```python
from build123d import *

# Parameters (mm, degrees)
F0_W      = 400
F0_H      = 500
F1_DEPTH  = 3
F2_W      = 10
F2_H      = 3
F2_W_2    = 20
F3_DEPTH  = 3
F4_W      = 20
F4_H      = 3
F5_DEPTH  = 3.001
F6_W      = 300
F6_H      = 300
F7_DEPTH  = 25
F8_R      = 25
F9_R      = 3
F10_DEPTH = 25


with BuildPart() as f1:
    # F0 (on Right) → F1 (new body)
    with BuildSketch(Plane.YZ):
        Rectangle(F0_W, F0_H)
    extrude(amount=F1_DEPTH)

    # F2 (on face) → F3 (join, through all)
    with BuildSketch(Plane.YZ.offset(3)):
        with Locations((-195, 251.5)):
            Rectangle(F2_W, F2_H)
        with Locations((-160, 251.5)):
            Rectangle(F2_W_2, F2_H)
        with Locations((-120, 251.5)):
            Rectangle(F2_W_2, F2_H)
        with Locations((-80, 251.5)):
            Rectangle(F2_W_2, F2_H)
        with Locations((-40, 251.5)):
            Rectangle(F2_W_2, F2_H)
        with Locations((0, 251.5)):
            Rectangle(F2_W_2, F2_H)
        with Locations((40, 251.5)):
            Rectangle(F2_W_2, F2_H)
        with Locations((80, 251.5)):
            Rectangle(F2_W_2, F2_H)
        with Locations((120, 251.5)):
            Rectangle(F2_W_2, F2_H)
        with Locations((160, 251.5)):
            Rectangle(F2_W_2, F2_H)
        with Locations((195, 251.5)):
            Rectangle(F2_W, F2_H)
        with Locations((-195, -251.5)):
            Rectangle(F2_W, F2_H)
        with Locations((-160, -251.5)):
            Rectangle(F2_W_2, F2_H)
        with Locations((-120, -251.5)):
            Rectangle(F2_W_2, F2_H)
        with Locations((195, -251.5)):
            Rectangle(F2_W, F2_H)
        with Locations((-80, -251.5)):
            Rectangle(F2_W_2, F2_H)
        with Locations((160, -251.5)):
            Rectangle(F2_W_2, F2_H)
        with Locations((0, -251.5)):
            Rectangle(F2_W_2, F2_H)
        with Locations((120, -251.5)):
            Rectangle(F2_W_2, F2_H)
        with Locations((-40, -251.5)):
            Rectangle(F2_W_2, F2_H)
        with Locations((40, -251.5)):
            Rectangle(F2_W_2, F2_H)
        with Locations((80, -251.5)):
            Rectangle(F2_W_2, F2_H)
    extrude(amount=-F3_DEPTH)

    # F4 (on face) → F5 (cut, through all)
    with BuildSketch(Plane(origin=(0, 0, 0), x_dir=(0, -1, 0), z_dir=(-1, 0, 0))):
        with Locations((-180, -151.5)):
            Rectangle(F4_W, F4_H)
        with Locations((-140, -151.5)):
            Rectangle(F4_W, F4_H)
        with Locations((-100, -151.5)):
            Rectangle(F4_W, F4_H)
        with Locations((-60, -151.5)):
            Rectangle(F4_W, F4_H)
        with Locations((-20, -151.5)):
            Rectangle(F4_W, F4_H)
        with Locations((20, -151.5)):
            Rectangle(F4_W, F4_H)
        with Locations((60, -151.5)):
            Rectangle(F4_W, F4_H)
        with Locations((100, -151.5)):
            Rectangle(F4_W, F4_H)
        with Locations((140, -151.5)):
            Rectangle(F4_W, F4_H)
        with Locations((180, -151.5)):
            Rectangle(F4_W, F4_H)
    extrude(amount=-F5_DEPTH, mode=Mode.SUBTRACT)

    # F6 (on face) → F7 (cut)
    with BuildSketch(Plane(origin=(0, 0, 0), x_dir=(0, -1, 0), z_dir=(-1, 0, 0))):
        with Locations((0, 51.5)):
            Rectangle(F6_W, F6_H)
    extrude(amount=-F7_DEPTH, mode=Mode.SUBTRACT)

    # F8
    f8_edges = [f1.edges().sort_by_distance(p)[0] for p in [
        (1.5, 150, 201.5),
        (1.5, -150, 201.5),
        (1.5, -150, -98.5),
        (1.5, 150, -98.5),
    ]]
    fillet(f8_edges, radius=F8_R)

    # F9 (on face) → F10 (cut)
    with BuildSketch(Plane.YZ.offset(3)):
        with Locations((0, 225.75)):
            Circle(F9_R)
        with Locations((-175, 51.5)):
            Circle(F9_R)
        with Locations((175, 51.5)):
            Circle(F9_R)
    extrude(amount=-F10_DEPTH, mode=Mode.SUBTRACT)


solid = f1.part
```
Could you check a few things on this model? Use its own coordinates, in mm. A direction names the side the tool comes from. Give positions to 0.01 mm unless a question says otherwise; leave off trailing zeros. Loops run counter-clockwise (first coordinate to the right, second up) from the corner with the lowest first, then second, coordinate; pieces in that order, holes last. Notation, with made-up numbers: (-1, 45.5) - (46, 45.5) arc R20 ccw to (46, 65.5) - close; hole circle Ø7 at (49.25, 39). An arc over 180 degrees is marked (long way). Answer in a Markdown table with one row per item. Add a question column.
Q1. Please list where these lines run through material, in increasing order: L1, parallel to Z at x = 2.6, y = 18.5; L2, parallel to Z at x = 1.6, y = 0; L3, parallel to Z at x = 0.25, y = -184. Write a range as from..to.
Q2. If we section it at B-B (z = -56.5): List the corners of the cut face in (x, y) for me.
Q3. For pin 1 (0.9 mm diameter, centred on x = 2, y = -136, fed in from +Z); pin 2 (0.9 mm diameter, centred on x = 1, y = -101, fed in from -Z); pin 3 (12 mm diameter, centred on y = -82, z = -136, fed in from -X), each with a flat end and sliding along its axis, tell me the tip position at first contact or that it passes through.
Q4. Which directions (+Z, -Z, +X, -X, +Y, -Y) give clear straight access to the entire face, cutting with the end or side of a thin tool? Please do faces 1 (the face through (0, -3, -109)), 2 (the face through (1.521, -142.482, 194.371)).
Q5. If we section it at C-C (x = 0.9): State how many separate pieces and enclosed holes the cut face has, plus the area to 3 significant figures.
Q6. We'd pull the mould along Y, two halves only. Please class faces 3 (the face through (1.521, -142.871, -90.982)), 4 (the face through (3, -3, -109)): +Y half, -Y half, draft (parallel to the pull), parting line (faces both ways), or undercut.
Q7. If we section it at A-A (y = -79.5): List the corners of the cut face in (x, z) for me, plus the area to 3 significant figures.
The answers:
| question | item | result |
|---|---|---|
| 1 | L1 | z = -250..-153, -150..-98.5, 201.5..250 |
| 1 | L2 | z = -253..-98.5, 201.5..222.75, 228.75..253 |
| 1 | L3 | z = -250..-153, -150..250 |
| 2 | outline | (0, -200) - (3, -200) - (3, -150) - (0, -150) - close; (0, 150) - (3, 150) - (3, 200) - (0, 200) - close |
| 3 | pin 1 | stops at z = 250 |
| 3 | pin 2 | stops at z = -250 |
| 3 | pin 3 | stops at x = 0 |
| 4 | face 1 | +Z, -Z, -X, +Y, -Y |
| 4 | face 2 | +X, -X |
| 5 | separate pieces | 1 |
| 5 | enclosed holes | 14 |
| 5 | area | 111,000 mm^2 |
| 6 | face 3 | undercut |
| 6 | face 4 | draft |
| 7 | outline | (0, -253) - (3, -253) - (3, -98.5) - (0, -98.5) - close; (0, 201.5) - (3, 201.5) - (3, 253) - (0, 253) - close |
| 7 | area | 618 mm^2 |
